Check sheet for the modelled part. Datum: model origin and axes. Units: mm. A direction names the side the tool comes from. Give positions to 0.01 mm unless a question says otherwise; leave off trailing zeros. Write each loop counter-clockwise with the first axis right and the second up, starting at its lowest first coordinate (ties: lowest second). Pieces come first, ordered by that corner, then holes. Notation, with made-up numbers: M 55,-37.5 L 90,-37.5 A27 cw 90,-11.5 Z; hole C -39.5,20 d9. An arc over 180 degrees is marked long. One line per item, written item: value. Start each with the question number.
from build123d import *

# Parameters (mm, degrees)
BOSS_EXTRU_1_DEPTH      = 6
ESQUISSE3_R             = 8
ESQUISSE3_W             = 6
ESQUISSE3_H             = 20
ESQUISSE3_W_2           = 20
ESQUISSE3_H_2           = 6
ESQUISSE3_W_3           = 60
ESQUISSE3_H_3           = 110
ESQUISSE3_W_4           = 8
ESQUISSE3_W_5           = 15
ESQUISSE3_H_4           = 29
ENL_V_MAT_EXTRU_2_DEPTH = 6
ESQUISSE4_R             = 1.5
ENL_V_MAT_EXTRU_3_DEPTH = 6
ESQUISSE5_W             = 456.045253014
ESQUISSE5_H             = 136.228984631
ENL_V_MAT_EXTRU_4_DEPTH = 6


with BuildPart() as part:
    # Esquisse1 → Boss.-Extru.1 (new body)
    with BuildSketch(Plane.XY):
        Polygon((-165, 96.73), (165, 96.73), (165, -18.27), (123, -109.022410436), (-123, -109.022410436), (-165, -18.27), align=None)
    extrude(amount=BOSS_EXTRU_1_DEPTH)

    # Esquisse3 → Enlèv. mat.-Extru.2 (cut)
    with BuildSketch(Plane(origin=(0, 0, 0), x_dir=(-1, 0, 0), z_dir=(0, 0, -1))):
        with Locations((130, -10.145)):
            Circle(ESQUISSE3_R)
        with Locations((162, 36.44)):
            Rectangle(ESQUISSE3_W, ESQUISSE3_H)
        with Locations((162, 72.73)):
            Rectangle(ESQUISSE3_W, ESQUISSE3_H)
        with Locations((162, 0.15)):
            Rectangle(ESQUISSE3_W, ESQUISSE3_H)
        with Locations((-30, -35.02)):
            Rectangle(ESQUISSE3_W_2, ESQUISSE3_H_2)
        with Locations((105, -35.02)):
            Rectangle(ESQUISSE3_W_2, ESQUISSE3_H_2)
        with Locations((-80, 29.355)):
            Rectangle(ESQUISSE3_W_3, ESQUISSE3_H_3)
        with Locations((-162, 72.73)):
            Rectangle(ESQUISSE3_W, ESQUISSE3_H)
        with Locations((30, -35.02)):
            Rectangle(ESQUISSE3_W_2, ESQUISSE3_H_2)
        with Locations((-162, 36.44)):
            Rectangle(ESQUISSE3_W, ESQUISSE3_H)
        with Locations((-162, 0.15)):
            Rectangle(ESQUISSE3_W, ESQUISSE3_H)
        with Locations((105, 93.73)):
            Rectangle(ESQUISSE3_W_2, ESQUISSE3_H_2)
        with Locations((-35, 93.73)):
            Rectangle(ESQUISSE3_W_2, ESQUISSE3_H_2)
        with Locations((35, 93.73)):
            Rectangle(ESQUISSE3_W_2, ESQUISSE3_H_2)
        with Locations((-105, 93.73)):
            Rectangle(ESQUISSE3_W_2, ESQUISSE3_H_2)
        with Locations((100.5, -10.145)):
            Rectangle(ESQUISSE3_W_4, ESQUISSE3_H)
        with Locations((-105, -35.02)):
            Rectangle(ESQUISSE3_W_2, ESQUISSE3_H_2)
        with Locations((71.5, -10.145)):
            Rectangle(ESQUISSE3_W_5, ESQUISSE3_H_4)
    extrude(amount=-ENL_V_MAT_EXTRU_2_DEPTH, mode=Mode.SUBTRACT)

    # Esquisse4 → Enlèv. mat.-Extru.3 (cut)
    with BuildSketch(Plane(origin=(0, 0, 0), x_dir=(-1, 0, 0), z_dir=(0, 0, -1))):
        with Locations(Location((162, 18.29, 0), (0, 0, 180))):
            Circle(ESQUISSE4_R)
        with Locations((120, -35.02)):
            Circle(ESQUISSE4_R)
        with Locations(Location((162, 54.585, 0), (0, 0, 180))):
            Circle(ESQUISSE4_R)
        with Locations((90, -35.02)):
            Circle(ESQUISSE4_R)
        with Locations((45, -35.02)):
            Circle(ESQUISSE4_R)
        with Locations((15, -35.02)):
            Circle(ESQUISSE4_R)
        with Locations(Location((-15, -35.02, 0), (0, 0, 180))):
            Circle(ESQUISSE4_R)
        with Locations(Location((-45, -35.02, 0), (0, 0, 180))):
            Circle(ESQUISSE4_R)
        with Locations(Location((-90, -35.02, 0), (0, 0, 180))):
            Circle(ESQUISSE4_R)
        with Locations((120, 93.73)):
            Circle(ESQUISSE4_R)
        with Locations(Location((-120, -35.02, 0), (0, 0, 180))):
            Circle(ESQUISSE4_R)
        with Locations((90, 93.73)):
            Circle(ESQUISSE4_R)
        with Locations((50, 93.73)):
            Circle(ESQUISSE4_R)
        with Locations((20, 93.73)):
            Circle(ESQUISSE4_R)
        with Locations((-162, 18.29)):
            Circle(ESQUISSE4_R)
        with Locations((-162, 54.585)):
            Circle(ESQUISSE4_R)
        with Locations(Location((-20, 93.73, 0), (0, 0, 180))):
            Circle(ESQUISSE4_R)
        with Locations(Location((-50, 93.73, 0), (0, 0, 180))):
            Circle(ESQUISSE4_R)
        with Locations(Location((-90, 93.73, 0), (0, 0, 180))):
            Circle(ESQUISSE4_R)
        with Locations(Location((-120, 93.73, 0), (0, 0, 180))):
            Circle(ESQUISSE4_R)
    extrude(amount=-ENL_V_MAT_EXTRU_3_DEPTH, mode=Mode.SUBTRACT)

    # Esquisse5 → Enlèv. mat.-Extru.4 (cut)
    with BuildSketch(Plane(origin=(0, 0, 0), x_dir=(-1, 0, 0), z_dir=(0, 0, -1))):
        with Locations((-18.307092018, -106.134492316)):
            Rectangle(ESQUISSE5_W, ESQUISSE5_H)
    extrude(amount=-ENL_V_MAT_EXTRU_4_DEPTH, mode=Mode.SUBTRACT)


solid = part.part
1) Tool access check on faces 1 (the flat face through (162, 26.44, 3)), 2 (the flat face through (35, 90.73, 3)), 3 (the flat face through (40, -35, 3)), 4 (the flat face through (110, 29, 3)). Record the directions out of +Z, -Z, +X, -X, +Y, -Y that give a thin tool (end or side, any length) a straight path to the whole face; none if there is none.
2) Cross-section at C-C (x = -30). Record the boundary of the cut face in (y, z), plus the area to 4 significant figures.
3) Draft check along Y on faces 5 (the flat face through (70, 96.73, 3)), 6 (the flat face through (-159, 0, 3)), 7 (the flat face through (-100, -0.145, 3)), 8 (the flat face through (-67, -38.02, 3)). Enter one of: released by +Y, released by -Y, zero draft, split by the parting line, or undercut.
4) Material ranges on L1, parallel to X at y = 0.5, z = 3.55; L2, parallel to Y at x = 105, z = 3.3 (3 decimals); L3, parallel to X at y = -21, z = 5.4, recorded low to high. Write a range as from..to.
5) Gauge pin test, flat ends, axial feed: pin 1 (3 mm diameter, centred on y = 75, z = 3, fed in from +X); pin 2 (1.8 mm diameter, centred on y = -35, z = 2.5, fed in from -X). Record the tip position at first contact, or that the pin passes through.
6) Cross-section at A-A (x = 75.5). Record the boundary of the cut face in (y, z) (3 decimals).
7) Cross-section at B-B (z = 2.8). State how many separate pieces and enclosed holes the cut face has, plus the area to 3 significant figures.
Data:
1. face 1: +Z, -Z, +X
1. face 2: +Z, -Z, +Y
1. face 3: +Z, -Z, -Y
1. face 4: +Z, -Z
2. outline: M -32.02,0 L 90.73,0 L 90.73,6 L -32.02,6 Z
2. area: 736.5 mm2
3. face 5: released by +Y
3. face 6: undercut
3. face 7: undercut
3. face 8: released by -Y
4. L1: x = -159..-79, -64..50, 110..159
4. L2: y = -32.02..-25.645, 84.355..90.73
4. L3: x = -163.74..-79, -64..50, 110..163.74
5. pin 1: stops at x = 159
5. pin 2: stops at x = -157.67
6. outline: M -38.02,0 L -25.645,0 L -25.645,6 L -38.02,6 Z; M 84.355,0 L 96.73,0 L 96.73,6 L 84.355,6 Z
7. separate pieces: 1
7. enclosed holes: 24
7. area: 35,100 mm2
